from build123d import *

# Parameters (mm, degrees)
CROQUIS1_W              = 50
CROQUIS1_H              = 110
SALIENTE_EXTRUIR1_DEPTH = 4.5
REDONDEO1_R             = 2
CROQUIS2_R              = 3.5
CROQUIS2_R_2            = 2.6
SALIENTE_EXTRUIR2_DEPTH = 5
CROQUIS3_W              = 35
CROQUIS3_H              = 90
SALIENTE_EXTRUIR3_DEPTH = 23
CROQUIS5_W              = 30
CROQUIS5_H              = 21
CORTAR_EXTRUIR2_DEPTH   = 106.61249926
CORTAR_EXTRUIR5_DEPTH   = 74.213728221
SALIENTE_EXTRUIR4_DEPTH = 5


with BuildPart() as part:
    # Croquis1 → Saliente-Extruir1 (new body)
    with BuildSketch(Plane.XY):
        Rectangle(CROQUIS1_W, CROQUIS1_H)
    extrude(amount=SALIENTE_EXTRUIR1_DEPTH)

    # Redondeo1
    redondeo1_edges = [part.edges().sort_by_distance(p)[0] for p in [
        (-25, 0, 4.5),
        (0, -55, 4.5),
        (25, 0, 4.5),
        (0, -55, 0),
        (-25, 0, 0),
        (0, 55, 0),
        (25, 0, 0),
        (0, 55, 4.5),
    ]]
    fillet(redondeo1_edges, radius=REDONDEO1_R)

    # Croquis2 → Saliente-Extruir2 (add)
    # profile 1 of 16: a face of its own
    with BuildSketch(Plane.XY.offset(4.5)):
        with Locations(Location((-15, 50, 0), (0, 0, 121.002719134))):
            Circle(CROQUIS2_R)
        with Locations((-15, 50)):
            Circle(CROQUIS2_R_2, mode=Mode.SUBTRACT)
    # profile 2 of 16: a face of its own
    with BuildSketch(Plane.XY.offset(4.5)):
        with Locations((-15, 40)):
            Circle(CROQUIS2_R)
        with Locations((-15, 40)):
            Circle(CROQUIS2_R_2, mode=Mode.SUBTRACT)
    # profile 3 of 16: a face of its own
    with BuildSketch(Plane.XY.offset(4.5)):
        with Locations((-9, 45)):
            Circle(CROQUIS2_R)
        with Locations((-9, 45)):
            Circle(CROQUIS2_R_2, mode=Mode.SUBTRACT)
    # profile 4 of 16: a face of its own
    with BuildSketch(Plane.XY.offset(4.5)):
        with Locations(Location((-21, 45, 0), (0, 0, 235.150095421))):
            Circle(CROQUIS2_R)
        with Locations(Location((-21, 45, 0), (0, 0, 219.715137232))):
            Circle(CROQUIS2_R_2, mode=Mode.SUBTRACT)
    # profile 5 of 16: a face of its own
    with BuildSketch(Plane.XY.offset(4.5)):
        with Locations(Location((21, 45, 0), (0, 0, 180))):
            Circle(CROQUIS2_R)
        with Locations(Location((21, 45, 0), (0, 0, 180))):
            Circle(CROQUIS2_R_2, mode=Mode.SUBTRACT)
    # profile 6 of 16: a face of its own
    with BuildSketch(Plane.XY.offset(4.5)):
        with Locations(Location((15, 40, 0), (0, 0, 180))):
            Circle(CROQUIS2_R)
        with Locations(Location((15, 40, 0), (0, 0, 180))):
            Circle(CROQUIS2_R_2, mode=Mode.SUBTRACT)
    # profile 7 of 16: a face of its own
    with BuildSketch(Plane.XY.offset(4.5)):
        with Locations(Location((9, 45, 0), (0, 0, 180))):
            Circle(CROQUIS2_R)
        with Locations(Location((9, 45, 0), (0, 0, 180))):
            Circle(CROQUIS2_R_2, mode=Mode.SUBTRACT)
    # profile 8 of 16: a face of its own
    with BuildSketch(Plane.XY.offset(4.5)):
        with Locations(Location((15, 50, 0), (0, 0, 180))):
            Circle(CROQUIS2_R)
        with Locations(Location((15, 50, 0), (0, 0, 180))):
            Circle(CROQUIS2_R_2, mode=Mode.SUBTRACT)
    # profile 9 of 16: a face of its own
    with BuildSketch(Plane.XY.offset(4.5)):
        with Locations((15, -40)):
            Circle(CROQUIS2_R)
        with Locations((15, -40)):
            Circle(CROQUIS2_R_2, mode=Mode.SUBTRACT)
    # profile 10 of 16: a face of its own
    with BuildSketch(Plane.XY.offset(4.5)):
        with Locations(Location((21, -45, 0), (0, 0, 55.150095421))):
            Circle(CROQUIS2_R)
        with Locations(Location((21, -45, 0), (0, 0, 39.715137232))):
            Circle(CROQUIS2_R_2, mode=Mode.SUBTRACT)
    # profile 11 of 16: a face of its own
    with BuildSketch(Plane.XY.offset(4.5)):
        with Locations((9, -45)):
            Circle(CROQUIS2_R)
        with Locations((9, -45)):
            Circle(CROQUIS2_R_2, mode=Mode.SUBTRACT)
    # profile 12 of 16: a face of its own
    with BuildSketch(Plane.XY.offset(4.5)):
        with Locations(Location((15, -50, 0), (0, 0, 238.997280866))):
            Circle(CROQUIS2_R)
        with Locations((15, -50)):
            Circle(CROQUIS2_R_2, mode=Mode.SUBTRACT)
    # profile 13 of 16: a face of its own
    with BuildSketch(Plane.XY.offset(4.5)):
        with Locations(Location((-15, -40, 0), (0, 0, 180))):
            Circle(CROQUIS2_R)
        with Locations(Location((-15, -40, 0), (0, 0, 180))):
            Circle(CROQUIS2_R_2, mode=Mode.SUBTRACT)
    # profile 14 of 16: a face of its own
    with BuildSketch(Plane.XY.offset(4.5)):
        with Locations(Location((-9, -45, 0), (0, 0, 180))):
            Circle(CROQUIS2_R)
        with Locations(Location((-9, -45, 0), (0, 0, 180))):
            Circle(CROQUIS2_R_2, mode=Mode.SUBTRACT)
    # profile 15 of 16: a face of its own
    with BuildSketch(Plane.XY.offset(4.5)):
        with Locations(Location((-21, -45, 0), (0, 0, 180))):
            Circle(CROQUIS2_R)
        with Locations(Location((-21, -45, 0), (0, 0, 180))):
            Circle(CROQUIS2_R_2, mode=Mode.SUBTRACT)
    # profile 16 of 16: a face of its own
    with BuildSketch(Plane.XY.offset(4.5)):
        with Locations(Location((-15, -50, 0), (0, 0, 180))):
            Circle(CROQUIS2_R)
        with Locations(Location((-15, -50, 0), (0, 0, 180))):
            Circle(CROQUIS2_R_2, mode=Mode.SUBTRACT)
    extrude(amount=SALIENTE_EXTRUIR2_DEPTH)

    # Croquis3 → Saliente-Extruir3 (add)
    with BuildSketch(Plane(origin=(0, 0, 0), x_dir=(-1, 0, 0), z_dir=(0, 0, -1))):
        Rectangle(CROQUIS3_W, CROQUIS3_H)
    extrude(amount=SALIENTE_EXTRUIR3_DEPTH)

    # Croquis5 → Cortar-Extruir2 (cut, through all)
    with BuildSketch(Plane(origin=(0, 45, 0), x_dir=(1, 0, 0), z_dir=(0, 1, 0))):
        with Locations((0, 11.5)):
            Rectangle(CROQUIS5_W, CROQUIS5_H)
    extrude(amount=-CORTAR_EXTRUIR2_DEPTH, mode=Mode.SUBTRACT)

    # Croquis8 → Cortar-Extruir5 (cut, through all)
    with BuildSketch(Plane(origin=(17.5, 0, 0), x_dir=(0, 0, -1), z_dir=(1, 0, 0))):
        with BuildLine():
            add(Edge.make_bspline(
                [(2.569348743, 40.716245485), (9.080503754, 18.53762373), (10.580801765, -9.48585487), (2.377628668, -42.298547258)],
                knots=[0, 0, 0, 0, 1, 1, 1, 1], degree=3))
            add(Edge.make_bspline(
                [(2.377628668, -42.298547258), (5.133604453, -15.937039747), (3.893375388, 16.552759214), (2.569348743, 40.716245485)],
                knots=[0, 0, 0, 0, 1, 1, 1, 1], degree=3))
        make_face()
        with BuildLine():
            add(Edge.make_bspline(
                [(20.430651257, 40.716245485), (13.919496246, 18.53762373), (12.419198235, -9.48585487), (20.622371332, -42.298547258)],
                knots=[0, 0, 0, 0, 1, 1, 1, 1], degree=3))
            add(Edge.make_bspline(
                [(20.622371332, -42.298547258), (17.866395547, -15.937039747), (19.106624612, 16.552759214), (20.430651257, 40.716245485)],
                knots=[0, 0, 0, 0, 1, 1, 1, 1], degree=3))
        make_face()
    extrude(amount=-CORTAR_EXTRUIR5_DEPTH, mode=Mode.SUBTRACT)

    # Croquis9 → Saliente-Extruir4 (add)
    with BuildSketch(Plane.XY.offset(4.5)):
        Polygon((-12.981572725, -15.774008449), (-11.3, -15.774008449), (-11.3, -18.6), (-8.618398116, -18.6), (-8.618398116, -19.949759238), (-12.981572725, -19.949759238), align=None)
        Polygon((-12.981572725, 19.949759238), (-12.981572725, 15.774008449), (-11.3, 15.774008449), (-11.3, 18.6), (-8.618398116, 18.6), (-8.618398116, 19.949759238), align=None)
        Polygon((12.981572725, 19.949759238), (12.981572725, 15.774008449), (11.3, 15.774008449), (11.3, 18.6), (8.618398116, 18.6), (8.618398116, 19.949759238), align=None)
        Polygon((8.618398116, -19.949759238), (12.981572725, -19.949759238), (12.981572725, -15.774008449), (11.3, -15.774008449), (11.3, -18.6), (8.618398116, -18.6), align=None)
    extrude(amount=SALIENTE_EXTRUIR4_DEPTH)


solid = part.part
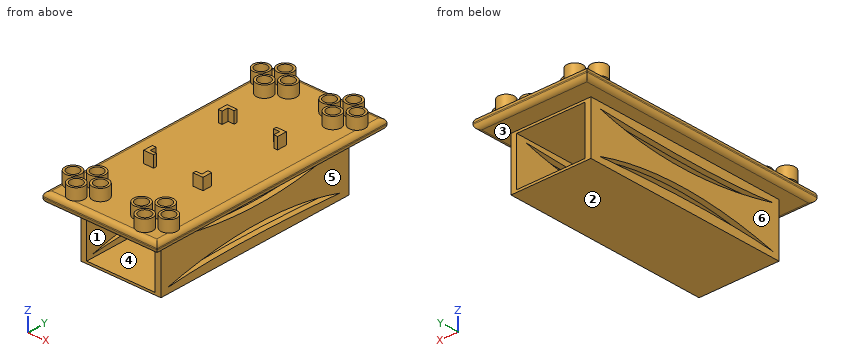
Input: part model. Units: mm. Frame: model coordinates. Face numbers are marked on the shaded views. A direction names the side the tool comes from. Round coordinates to 2 decimals unless told otherwise and drop trailing zeros. Loops run counter-clockwise (first coordinate to the right, second up) from the corner with the lowest first, then second, coordinate; pieces in that order, holes last. Notation, with made-up numbers: (-11, 22) -> (21, 22) arc R20 ccw to (21, 50) -> close; hole circle Ø3 at (22.25, 7). An arc over 180 degrees is marked (long way). Answer as a JSON object with one key per item and string values. Group by question number.
1) Section query D-D on x = -21. Output: boundary loops of the cut face in (y, z), plus the area to 3 significant figures.
2) Reachability of the marked faces 1 and 2 from +Z, -Z, +X, -X, +Y, -Y: full face, straight path, thin tool, end or side. Return the list, or none.
3) Pin query (flat end, axial travel): pin 1 (1.5 mm diameter, centred on x = 18, z = -8, fed in from +Y); pin 2 (18.5 mm diameter, centred on x = -4, z = -8.5, fed in from -Y); pin 3 (4 mm diameter, centred on x = -15.5, y = 50, fed in from +Z); pin 4 (12 mm diameter, centred on x = 6.5, z = -15, fed in from -Y). Return the tip coordinate at first contact, or that it passes through.
4) Section query A-A on z = -10. Output: boundary loops of the cut face in (x, y), plus the area to 3 significant figures.
5) Draft query along X for the marked faces 3, 4, 5 and 6. Return one class per face: +X half, -X half, draft (parallel to the pull), parting line (faces both ways), or undercut.
6) Ray query, L1, parallel to Y at x = -21, z = 5; L2, parallel to Z at x = -3, y = -34.5; L3, parallel to X at y = -27, z = -15. Return the intervals inside material, ascending.
7) Section query B-B on y = -50. Output: boundary loops of the cut face in (x, z), plus the area to 3 significant figures.
Reply:
{
 "1": {"outline": "(-55, 2) arc R2 ccw to (-53, 0) -> (53, 0) arc R2 ccw to (55, 2) -> (55, 2.5) arc R2 ccw to (53, 4.5) -> (48.5, 4.5) -> (48.5, 9.5) -> (47.6, 9.5) -> (47.6, 4.5) -> (42.4, 4.5) -> (42.4, 9.5) -> (41.5, 9.5) -> (41.5, 4.5) -> (-41.5, 4.5) -> (-41.5, 9.5) -> (-42.4, 9.5) -> (-42.4, 4.5) -> (-47.6, 4.5) -> (-47.6, 9.5) -> (-48.5, 9.5) -> (-48.5, 4.5) -> (-53, 4.5) arc R2 ccw to (-55, 2.5) -> close", "area": "510 mm2"},
 "2": {"face 1": "+Y, -Y", "face 2": "-Z, +X, -X, +Y, -Y"},
 "3": {"pin 1": "stops at y = 45", "pin 2": "stops at y = -54.56", "pin 3": "stops at z = 4.5", "pin 4": "passes through"},
 "4": {"outline": "(-17.5, -45) -> (-15, -45) -> (-15, 45) -> (-17.5, 45) -> close; (15, -45) -> (17.5, -45) -> (17.5, 45) -> (15, 45) -> close", "area": "450 mm2"},
 "5": {"face 3": "draft", "face 4": "undercut", "face 5": "+X half", "face 6": "-X half"},
 "6": {"L1": "y = -48.5 to -47.6, -42.4 to -41.5, 41.5 to 42.4, 47.6 to 48.5", "L2": "z = -23 to -22, -1 to 4.5", "L3": "x = -17.5 to -15, 15 to 17.5"},
 "7": {"outline": "(-25, 2) arc R2 ccw to (-23, 0) -> (23, 0) arc R2 ccw to (25, 2) -> (25, 2.5) arc R2 ccw to (23, 4.5) -> (18.5, 4.5) -> (18.5, 9.5) -> (17.6, 9.5) -> (17.6, 4.5) -> (12.4, 4.5) -> (12.4, 9.5) -> (11.5, 9.5) -> (11.5, 4.5) -> (-11.5, 4.5) -> (-11.5, 9.5) -> (-12.4, 9.5) -> (-12.4, 4.5) -> (-17.6, 4.5) -> (-17.6, 9.5) -> (-18.5, 9.5) -> (-18.5, 4.5) -> (-23, 4.5) arc R2 ccw to (-25, 2.5) -> close", "area": "240 mm2"}
}
